For this review, take the finished solid that the model builds, in its own axes (mm). A direction names the side the tool comes from. Give positions to 0.01 mm unless a question says otherwise; leave off trailing zeros. Order: outer loops, then holes, each group sorted by start corner. A loop starts at its lowest first (then second) coordinate and runs counter-clockwise, first axis right, second up. Notation, with made-up numbers: M 67,27 L 83,27 A12 cw 83,35 Z; hole C 41.25,85.5 d9. An arc over 180 degrees is marked long. Answer as CSV lines item,"result". Start each with the question number.
1. We need section D-D, the plane y = 14. Give the boundary of the cut face in (x, z), and give its area (3 significant figures).
2. Mouldability with a two-part tool opening along Z and no side actions: class faces 1 (the flat face through (0, -5, 0)), 2 (the cylindrical face through (2.535, 12.493, -18.713)), 3 (the cylindrical face through (2.465, 11.945, 11.919)), 4 (the cylindrical face through (2.535, 18.713, 12.493)) as pulls with the +Z half, pulls with the -Z half, needs draft (parallel to the pull), parting line crosses it, or undercut.
3. Machinability: for faces 5 (the cylindrical face through (2.465, 17.485, -9.471)), 6 (the cylindrical face through (2.535, -22.066, 4.398)), 7 (the cylindrical face through (2.465, 9.471, 17.485)), 8 (the cylindrical face through (2.465, -11.945, -11.919)), 9 (the cylindrical face through (2.465, -19.702, -2.023)), which of the approach directions +Z, -Z, +X, -X, +Y, -Y give a long, thin tool a straight path to every point of the face, cutting with its end or side? Answer none if there is none.
4. Clearance check with flat-ended pins moving along their axes: P1, Ø1.8, axis at y = 0.67, z = -6.97, coming from the -X side; P2, Ø3.5, axis at y = -0.67, z = 6.97, coming from the +X side; P3, Ø1.5, axis at x = 2.5, z = -17.5, coming from the +Y side. State where each tip first meets the part, or that it passes through.
5. We need section B-B, the plane z = 0. Give the boundary of the cut face in (x, y).
6. We need section A-A, the plane y = 0. Give the boundary of the cut face in (x, z).
7. For line 1 along Z through (x, y) = (3.95, -12); line 2 along Y through (x, z) = (1.6, 16.5); line 3 along Z through (x, y) = (2.2, -17) (3 decimals), list the stretches that pass through material, from the lowest coordinate up.
8. We need section C-C, the plane x = 1.4. State how many separate pieces and enclosed holes the cut face has, and give its area (3 significant figures).
from build123d import *

# Parameters (mm, degrees)
BASPROSKE_W             = 5
BASPROSKE_H             = 22.5
TOOTHCUT_DEPTH          = 33.210246817
TEETHCUTS_COUNT         = 16
TEETHCUTS_ANGLE         = 337.5
BORSKE_R                = 2.5
BORE_DEPTH              = 50.0000508
ESQUISSE1_R             = 9.9
ENL_V_MAT_EXTRU_1_DEPTH = 2
ESQUISSE2_R             = 1.5
ESQUISSE2_R_2           = 1.531300803
ENL_V_MAT_EXTRU_2_DEPTH = 32.503631705


with BuildPart() as part:
    # BasProSke → Base-Revolve (revolve)
    with BuildSketch(Plane(origin=(0, 0, 0), x_dir=(1, 0, 0), z_dir=(0, 1, 0)), mode=Mode.PRIVATE) as base_revolve_sk:
        with Locations((2.5, 11.25)):
            Rectangle(BASPROSKE_W, BASPROSKE_H)
    revolve(base_revolve_sk.sketch.rotate(Axis((-10, 0, 0), (1, 0, 0)), 180), axis=Axis((-10, 0, 0), (1, 0, 0)))

    # TooCutSke → ToothCut (cut, through all)
    with BuildSketch(Plane(origin=(0, 0, 0), x_dir=(0, 0, -1), z_dir=(1, 0, 0))):
        with BuildLine():
            ThreePointArc((1.297749273, 16.824022195), (0, 16.874), (-1.297749273, 16.824022195))
            ThreePointArc((-1.297749273, 16.824022195), (-2.047921493, 19.754510488), (-3.832565589, 22.196961192))
            ThreePointArc((-3.832565589, 22.196961192), (0, 22.5254), (3.832565589, 22.196961192))
            ThreePointArc((3.832565589, 22.196961192), (2.047921493, 19.754510488), (1.297749273, 16.824022195))
        make_face()
    toothcut = extrude(amount=TOOTHCUT_DEPTH, mode=Mode.SUBTRACT)

    # TeethCuts: ToothCut ×16 about axis
    teethcuts_axis = Axis((-10, 0, 0), (1, 0, 0))
    for i in range(1, TEETHCUTS_COUNT):
        add(toothcut.rotate(teethcuts_axis, i * TEETHCUTS_ANGLE / (TEETHCUTS_COUNT - 1)), mode=Mode.SUBTRACT)

    # BorSke → Bore (cut, symmetric)
    with BuildSketch(Plane(origin=(0, 0, 0), x_dir=(0, 0, -1), z_dir=(1, 0, 0))):
        with Locations(Location((0, 0, 0), (0, 0, 180))):
            Circle(BORSKE_R)
    extrude(amount=BORE_DEPTH, both=True, mode=Mode.SUBTRACT)

    # Esquisse1 → Enlèv. mat.-Extru.1 (cut)
    with BuildSketch(Plane(origin=(5, 0, 0), x_dir=(0, 0, -1), z_dir=(1, 0, 0))):
        Circle(ESQUISSE1_R)
    extrude(amount=-ENL_V_MAT_EXTRU_1_DEPTH, mode=Mode.SUBTRACT)

    # Esquisse2 → Enlèv. mat.-Extru.2 (cut, through all)
    with BuildSketch(Plane(origin=(3, 0, 0), x_dir=(0, 0, -1), z_dir=(1, 0, 0))):
        with Locations((-0.665922194, 6.968252839)):
            Circle(ESQUISSE2_R)
        with Locations((6.968252839, 0.665922194)):
            Circle(ESQUISSE2_R_2)
        with Locations((0.665922194, -6.968252839)):
            Circle(ESQUISSE2_R)
        with Locations((-6.968252839, -0.665922194)):
            Circle(ESQUISSE2_R)
    extrude(amount=-ENL_V_MAT_EXTRU_2_DEPTH, mode=Mode.SUBTRACT)


solid = part.part
Result set:
1,outline,"M 0,-11.85 L 5,-11.85 L 5,11.85 L 0,11.85 Z"
1,area,"118 mm2"
2,face 1,"needs draft"
2,face 2,"pulls with the -Z half"
2,face 3,"undercut"
2,face 4,"pulls with the +Z half"
3,face 5,"+X, -X, +Y"
3,face 6,"+Z, +X, -X, -Y"
3,face 7,"+Z, +X, -X"
3,face 8,"+X, -X"
3,face 9,"+X, -X, -Y"
4,P1,"through"
4,P2,"x = 3"
4,P3,"y = 12.99"
5,outline,"M 0,-16.87 L 5,-16.87 L 5,-9.9 L 3,-9.9 L 3,-8.31 L 0,-8.31 Z; M 0,-5.62 L 3,-5.62 L 3,-2.5 L 0,-2.5 Z; M 0,2.5 L 3,2.5 L 3,5.62 L 0,5.62 Z; M 0,8.31 L 3,8.31 L 3,9.9 L 5,9.9 L 5,16.87 L 0,16.87 Z"
6,outline,"M 0,-16.87 L 5,-16.87 L 5,-9.9 L 3,-9.9 L 3,-8.35 L 0,-8.35 Z; M 0,-5.59 L 3,-5.59 L 3,-2.5 L 0,-2.5 Z; M 0,2.5 L 3,2.5 L 3,5.62 L 0,5.62 Z; M 0,8.31 L 3,8.31 L 3,9.9 L 5,9.9 L 5,16.87 L 0,16.87 Z"
7,line 1,"-19.03 to -14.26, -11.86 to 11.86, 14.26 to 19.03"
7,line 2,"-12.83 to -8.55, -5.38 to 5.38, 8.55 to 12.83"
7,line 3,"-12.912 to -8.979, -5.505 to -1.31, 1.31 to 5.505, 8.979 to 12.912"
8,separate pieces,"1"
8,enclosed holes,"5"
8,area,"1,150 mm2"
